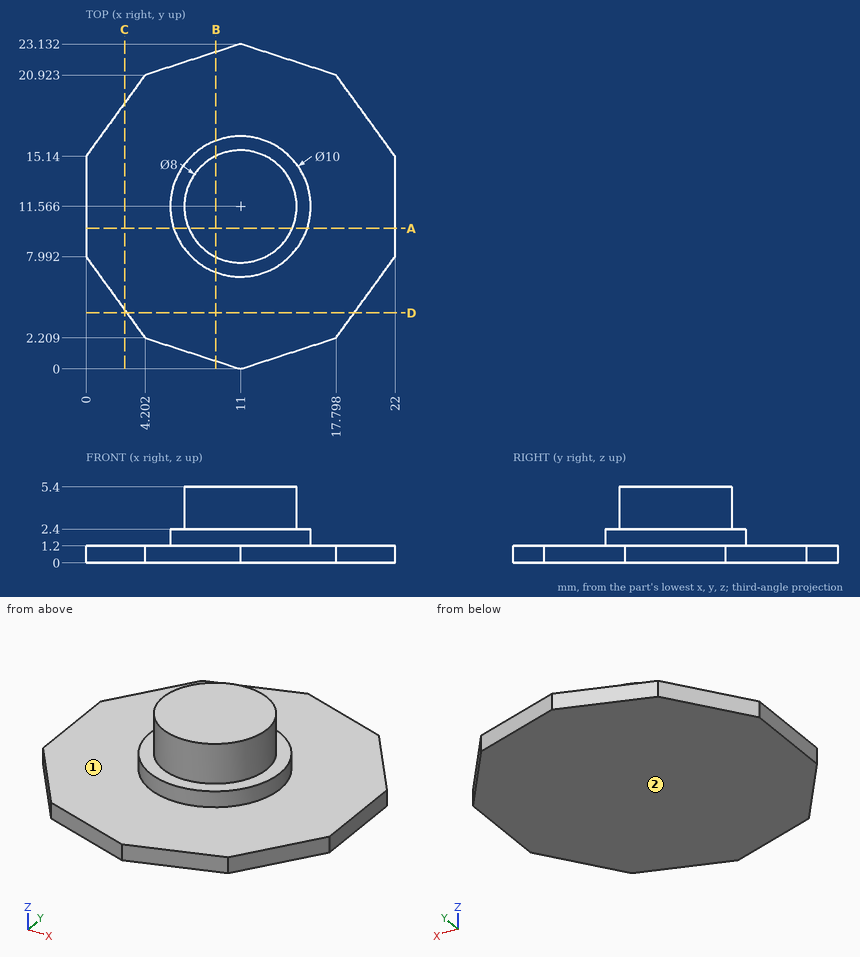
Here's the drawing with two shaded views (mm, measured from the low corner). I have some questions. A direction names the side the tool comes from. Give positions to 0.01 mm unless a question says otherwise; leave off trailing zeros. Write each loop counter-clockwise with the first axis right and the second up, starting at its lowest first coordinate (ties: lowest second). Pieces come first, ordered by that corner, then holes. Notation, with made-up numbers: (-38.75, 75) -> (-3.75, 75) arc R25 cw to (-3.75, 109) -> close; hole circle Ø1 at (43.5, -9). An arc over 180 degrees is marked (long way). Use one line per item in the form item = value. Start each with the question number.
1. Imagine slicing it at D-D on y = 4. List the corners of the cut face in (x, z) for me.
2. If I drill on L1, parallel to Z at x = 15.25, y = 20; L2, parallel to X at y = 19.5, z = 0.4; L3, parallel to Y at x = 12.75, z = 4.6, over which ranges is the centre line in solid material (lowest first)?
3. Will these pins go through, and if not, where does the flat tip stop? pin 1 Ø2 at (y, z) = (17, 1) entering from -X (1 decimal); pin 2 Ø12 at (x, y) = (13.5, 4) entering from +Z; pin 3 Ø5 at (x, y) = (19.5, 5) entering from +Z.
4. Imagine slicing it at A-A on y = 10. List the corners of the cut face in (x, z) for me.
5. Imagine slicing it at B-B on x = 9.25. List the corners of the cut face in (y, z) for me.
6. Imagine slicing it at C-C on x = 2.75. List the corners of the cut face in (y, z) for me (1 decimal).
7. On a 3-axis mill with a long thin cutter (end or side, diameter ignored), from which of +Z, -Z, +X, -X, +Y, -Y can I reach the whole of each face in a straight line? I mean the marked faces 1 and 2. Say none if no direction works.
Entries:
q1.outline = (2.9, 0) -> (19.1, 0) -> (19.1, 1.2) -> (2.9, 1.2) -> close
q2.L1 = 0 to 1.2
q2.L2 = 3.17 to 18.83
q2.L3 = 7.97 to 15.16
q3.pin_1 = 0.6
q3.pin_2 = 5.4
q3.pin_3 = 1.2
q4.outline = (0, 0) -> (22, 0) -> (22, 1.2) -> (15.75, 1.2) -> (15.75, 2.4) -> (14.68, 2.4) -> (14.68, 5.4) -> (7.32, 5.4) -> (7.32, 2.4) -> (6.25, 2.4) -> (6.25, 1.2) -> (0, 1.2) -> close
q5.outline = (0.57, 0) -> (22.56, 0) -> (22.56, 1.2) -> (16.25, 1.2) -> (16.25, 2.4) -> (15.16, 2.4) -> (15.16, 5.4) -> (7.97, 5.4) -> (7.97, 2.4) -> (6.88, 2.4) -> (6.88, 1.2) -> (0.57, 1.2) -> close
q6.outline = (4.2, 0) -> (18.9, 0) -> (18.9, 1.2) -> (4.2, 1.2) -> close
q7.face_1 = +Z
q7.face_2 = -Z, +X, -X, +Y, -Y
